```python
from build123d import *

# Parameters (mm, degrees)
F0_R     = 5
F1_DEPTH = 25
F3_D     = 6
F5_D     = 18


with BuildPart() as f1:
    # F0 (on Front) → F1 (new body)
    with BuildSketch(Plane.XZ):
        with BuildLine():
            ThreePointArc((22.737747, 27.324713), (20.562966, 2.515353), (18.388185, 27.324713))
            Line((18.388185, 27.324713), (18.388185, 39.324713))
            Line((18.388185, 39.324713), (-14.437034, 39.324713))
            Line((-14.437034, 39.324713), (-14.437034, -24.675287))
            Line((-14.437034, -24.675287), (20.562966, -24.675287))
            Line((20.562966, -24.675287), (55.562966, -24.675287))
            Line((55.562966, -24.675287), (55.562966, 39.324713))
            Line((55.562966, 39.324713), (22.737747, 39.324713))
            Line((22.737747, 39.324713), (22.737747, 27.324713))
        make_face()
        with Locations((41.062966, 15.015353)):
            Circle(F0_R, mode=Mode.SUBTRACT)
    extrude(amount=F1_DEPTH)

    # F3 (through all)
    with Locations(Plane(origin=(-14.437034, 0, 0), x_dir=(0, -1, 0), z_dir=(-1, 0, 0))):
        with Locations((12.5, 33.046592)):
            Hole(F3_D / 2)

    # F5 (through all)
    with Locations(Plane.YZ.offset(55.562966)):
        with Locations((-12.5, -12.675287)):
            Hole(F5_D / 2)


solid = f1.part
```
Check sheet for the modelled part. Datum: model origin and axes. Units: mm. A direction names the side the tool comes from. Round coordinates to 2 decimals unless told otherwise and drop trailing zeros. Loops run counter-clockwise (first coordinate to the right, second up) from the corner with the lowest first, then second, coordinate; pieces in that order, holes last. Notation, with made-up numbers: (-2, 30) -> (29, 30) arc R25 cw to (29, 52) -> close; hole circle Ø9 at (16.5, 47.5). An arc over 180 degrees is marked (long way). Answer in a Markdown table with one row per item.
Q1. Sectioned sample at C-C on x = 26.5. Enter the section's corners in (y, z), then the cut area to 3 significant figures.
Data:
| item | result |
|---|---|
| outline | (-25, -24.68) -> (0, -24.68) -> (0, 4.02) -> (-25, 4.02) -> close; (-25, 26.02) -> (0, 26.02) -> (0, 39.32) -> (-25, 39.32) -> close; hole circle Ø18 at (-12.5, -12.68); hole circle Ø6 at (-12.5, 33.05) |
| area | 767 mm^2 |
Q2. Set-up check for faces 1 (the face through (22.738, -10, 35)), 2 (the face through (45.68, -12.32, 13.1)): record each of +Z, -Z, +X, -X, +Y, -Y from which the full face is reachable in a straight line by a thin tool's end or side.
Data:
| item | result |
|---|---|
| face 1 | +Z, +Y, -Y |
| face 2 | +Y, -Y |
Q3. Sectioned sample at D-D on y = -6. Enter the section's corners in (x, z).
Data:
| item | result |
|---|---|
| outline | (-14.44, -24.68) -> (55.56, -24.68) -> (55.56, -18.9) -> (-14.44, -18.9) -> close; (-14.44, -6.45) -> (55.56, -6.45) -> (55.56, 39.32) -> (22.74, 39.32) -> (22.74, 27.32) arc R12.5 cw (long way) to (18.39, 27.32) -> (18.39, 39.32) -> (-14.44, 39.32) -> close; hole circle Ø10 at (41.06, 15.02) |
Q4. Go/stop test with a flat-tipped pin: P1, Ø5, axis at y = -12.5, z = 33.05, coming from the +X side. Record where the tip stops, or that it passes through.
Data:
| item | result |
|---|---|
| P1 | passes through |
Q5. Sectioned sample at A-A on y = -12.5. Enter the section's corners in (x, z).
Data:
| item | result |
|---|---|
| outline | (-14.44, -24.68) -> (55.56, -24.68) -> (55.56, -21.68) -> (-14.44, -21.68) -> close; (-14.44, -3.68) -> (55.56, -3.68) -> (55.56, 30.05) -> (22.74, 30.05) -> (22.74, 27.32) arc R12.5 cw (long way) to (18.39, 27.32) -> (18.39, 30.05) -> (-14.44, 30.05) -> close; (-14.44, 36.05) -> (18.39, 36.05) -> (18.39, 39.32) -> (-14.44, 39.32) -> close; (22.74, 36.05) -> (55.56, 36.05) -> (55.56, 39.32) -> (22.74, 39.32) -> close; hole circle Ø10 at (41.06, 15.02) |
Q6. Thickness scan on L1, parallel to Z at x = 3, y = -12.5; L2, parallel to X at y = -5, z = 36; L3, parallel to Z at x = 41, y = -22.5. Record the ranges inside material, lowest first.
Data:
| item | result |
|---|---|
| L1 | z = -24.68 to -21.68, -3.68 to 30.05, 36.05 to 39.32 |
| L2 | x = -14.44 to 18.39, 22.74 to 55.56 |
| L3 | z = -24.68 to 10.02, 20.01 to 39.32 |
Q7. Release check for a two-part mould opening along Y. For faces 3 (the face through (2, -12, 39.325)), 4 (the face through (20, -25, 1)), 5 (the face through (2.205, -14.711, 35.074)) record: released by +Y, released by -Y, zero draft, split by the parting line, or undercut.
Data:
| item | result |
|---|---|
| face 3 | zero draft |
| face 4 | released by -Y |
| face 5 | undercut |
Q8. Sectioned sample at B-B on z = -5. Enter the section's corners in (x, y).
Data:
| item | result |
|---|---|
| outline | (-14.44, -25) -> (55.56, -25) -> (55.56, -17.2) -> (-14.44, -17.2) -> close; (-14.44, -7.8) -> (55.56, -7.8) -> (55.56, 0) -> (-14.44, 0) -> close |
